Can you work these out from the drawing? Everything is in mm from the part's minimum corner. A direction names the side the tool comes from. Give positions to 0.01 mm unless a question says otherwise; leave off trailing zeros. Write each loop counter-clockwise with the first axis right and the second up, starting at its lowest first coordinate (ties: lowest second). Pieces come first, ordered by that corner, then holes. Notation, with made-up numbers: (-22.75, 52) -> (29.25, 52) arc R30 cw to (29.25, 75) -> close; hole circle Ø3 at (51, -18). An arc over 180 degrees is marked (long way). Use one line per item in the form item = value.
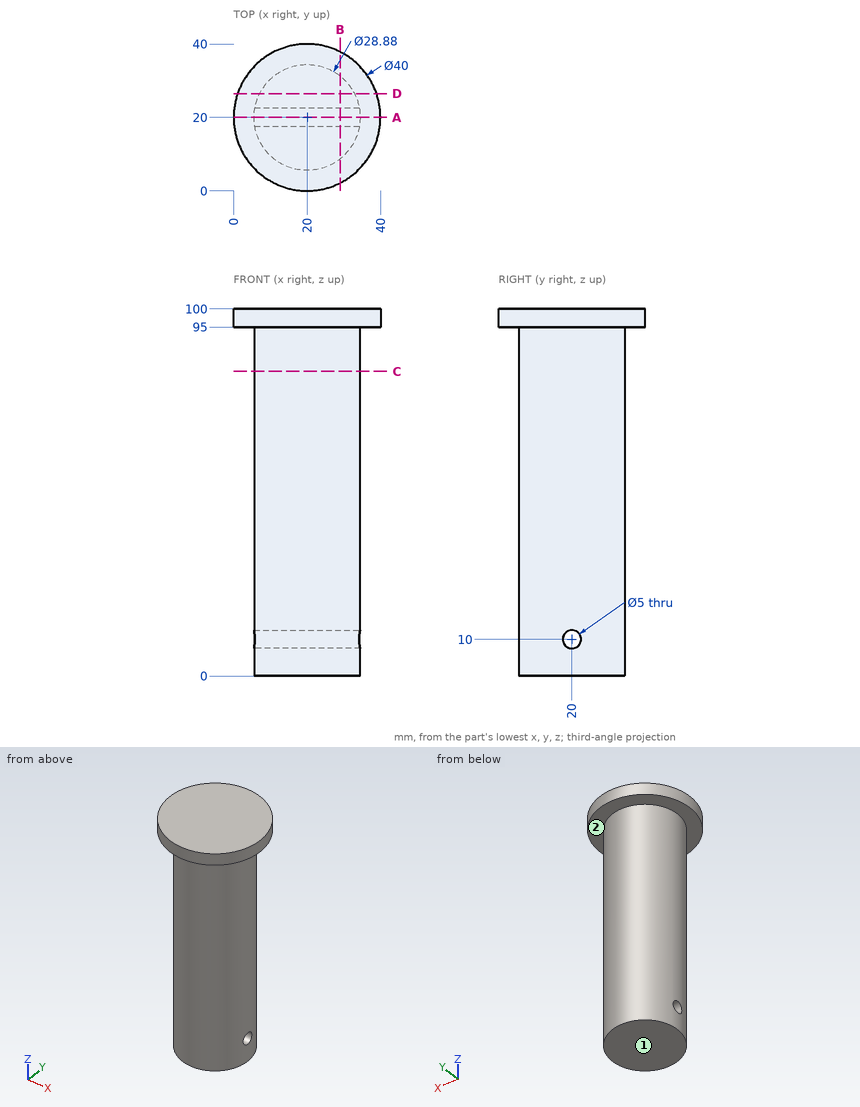
Q1. Will these pins go through, and if not, where does the flat tip stop? pin 1 Ø2 at (x, y) = (5.5, 15.5) entering from -Z; pin 2 Ø1 at (y, z) = (23, 12) entering from -X; pin 3 Ø10 at (x, z) = (9.5, 42) entering from -Y; pin 4 Ø2 at (y, z) = (28.5, 29.5) entering from -X.
Result set:
pin_1 = 0
pin_2 = 5.78
pin_3 = 6.65
pin_4 = 7.66
Q2. Which directions (+Z, -Z, +X, -X, +Y, -Y) give clear straight access to the entire face, cutting with the end or side of a thin tool? Please do the marked faces 1 and 2.
Result set:
face_1 = -Z, +X, -X, +Y, -Y
face_2 = -Z
Q3. I want a section at B-B, the plane x = 29. Write out the boundary of the cut face in (y, z).
Result set:
outline = (2.14, 95) -> (8.71, 95) -> (8.71, 0) -> (31.29, 0) -> (31.29, 95) -> (37.86, 95) -> (37.86, 100) -> (2.14, 100) -> close; hole circle Ø5 at (20, 10)
Q4. I want a section at C-C, the plane z = 83. Write out the boundary of the cut face in (x, y), and give its area (3 significant figures).
Result set:
outline = circle Ø28.88 at (20, 20)
area = 655 mm2
Q5. If I drill on line 1 along Y through (x, z) = (20.75, 10); line 2 along Z through (x, y) = (26, 20); line 3 along X through (y, z) = (19.5, 49), over which ranges is the centre line in solid material (lowest first)? Write a range as from..to.
Result set:
line_1 = 5.58..17.5, 22.5..34.42
line_2 = 0..7.5, 12.5..100
line_3 = 5.57..34.43
Q6. I want a section at D-D, the plane y = 26.5. Write out the boundary of the cut face in (x, z).
Result set:
outline = (1.09, 95) -> (7.11, 95) -> (7.11, 0) -> (32.89, 0) -> (32.89, 95) -> (38.91, 95) -> (38.91, 100) -> (1.09, 100) -> close
Q7. I want a section at A-A, the plane y = 20. Write out the boundary of the cut face in (x, z), and give its area (3 significant figures).
Result set:
outline = (0, 95) -> (5.56, 95) -> (5.56, 12.5) -> (34.44, 12.5) -> (34.44, 95) -> (40, 95) -> (40, 100) -> (0, 100) -> close; (5.56, 0) -> (34.44, 0) -> (34.44, 7.5) -> (5.56, 7.5) -> close
area = 2,800 mm2
